Here's the drawing with two shaded views (mm, measured from the low corner). I have some questions. Give positions to 0.01 mm unless a question says otherwise; leave off trailing zeros. Loops run counter-clockwise (first coordinate to the right, second up) from the corner with the lowest first, then second, coordinate; pieces in that order, holes last. Notation, with made-up numbers: (53, -25) - (77, -25) arc R17 cw to (77, -1) - close; hole circle Ø5 at (49, 5.25). An arc over 180 degrees is marked (long way). Answer as a JSON object with one key per item and string values. Group by question number.
Item 1: Suppose I cut it at B-B on y = 40.35. Write out the boundary of the cut face in (x, z).
Item 2: Suppose I cut it at D-D on y = 10.5. Write out the boundary of the cut face in (x, z).
Item 3: Suppose I cut it at A-A on x = 49. Write out the boundary of the cut face in (y, z).
Item 4: Thinking about a two-plate mould opening in X: for the marked faces 1 and 2, which applies, pulls with the +X half, pulls with the -X half, needs draft (parallel to the pull), parting line crosses it, or undercut?
Item 5: Suppose I cut it at C-C on z = 6. Write out the boundary of the cut face in (x, y), and give its area (3 significant figures).
Item 6: Please list where these lines run through material, in increasing order: L1, parallel to Y at x = 20, z = 9.5; L2, parallel to Y at x = 49, z = 5; L3, parallel to Z at x = 34, y = 39.5.
Item 7: Will these pins go through, and if not, where does the flat tip stop? pin 1 (4.5 mm diameter, centred on x = 20, y = 35, fed in from +Z); pin 2 (1.6 mm diameter, centred on x = 26.5, z = 2.5, fed in from +Y); pin 3 (5 mm diameter, centred on x = 33.5, z = 5.5, fed in from +Y); pin 4 (1 mm diameter, centred on x = 48.5, z = 13, fed in from +Y).
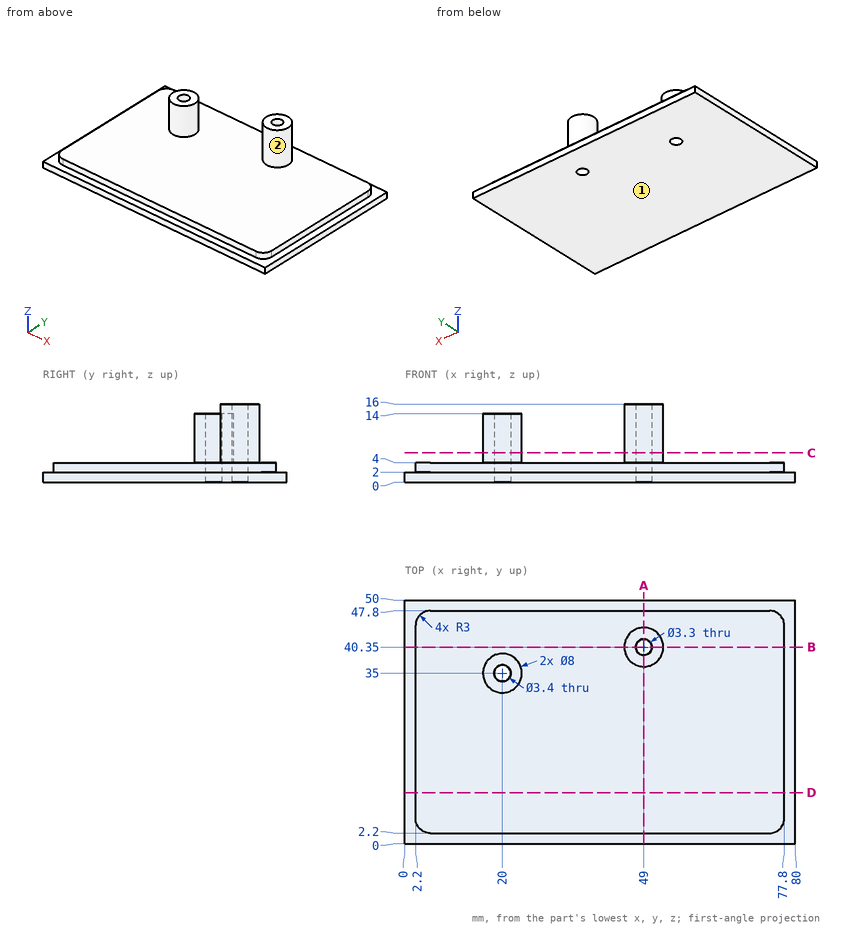
Worked out:
{
 "1": {"outline": "(0, 0) - (47.35, 0) - (47.35, 16) - (45, 16) - (45, 4) - (2.2, 4) - (2.2, 2) - (0, 2) - close; (50.65, 0) - (80, 0) - (80, 2) - (77.8, 2) - (77.8, 4) - (53, 4) - (53, 16) - (50.65, 16) - close"},
 "2": {"outline": "(0, 0) - (80, 0) - (80, 2) - (77.8, 2) - (77.8, 4) - (2.2, 4) - (2.2, 2) - (0, 2) - close"},
 "3": {"outline": "(0, 0) - (38.7, 0) - (38.7, 16) - (36.35, 16) - (36.35, 4) - (2.2, 4) - (2.2, 2) - (0, 2) - close; (42, 0) - (50, 0) - (50, 2) - (47.8, 2) - (47.8, 4) - (44.35, 4) - (44.35, 16) - (42, 16) - close"},
 "4": {"face 1": "needs draft", "face 2": "undercut"},
 "5": {"outline": "circle Ø8 at (20, 35); circle Ø8 at (49, 40.35); hole circle Ø3.4 at (20, 35); hole circle Ø3.3 at (49, 40.35)", "area": "82.9 mm2"},
 "6": {"L1": "y = 31 to 33.3, 36.7 to 39", "L2": "y = 36.35 to 38.7, 42 to 44.35", "L3": "z = 0 to 4"},
 "7": {"pin 1": "stops at z = 14", "pin 2": "stops at y = 50", "pin 3": "stops at y = 47.8", "pin 4": "stops at y = 44.35"}
}
